Can you work these out from the model? Positions are in its coordinate system, mm. Give positions to 0.01 mm unless a question says otherwise; leave off trailing zeros. Write each loop counter-clockwise with the first axis right and the second up, starting at its lowest first coordinate (ties: lowest second). Pieces come first, ordered by that corner, then holes.
1. I'm going to push flat-ended pins straight in: pin 1 (1 mm diameter, centred on x = -2, y = 93, fed in from +Z); pin 2 (3 mm diameter, centred on x = -0.5, z = -43, fed in from +Y); pin 3 (2.5 mm diameter, centred on y = 149.03, z = 29.78, fed in from -X); pin 4 (3 mm diameter, centred on x = -1.5, y = 119, fed in from -Z). Where does each tip first touch, or does it pass through?
2. Suppose I cut it at B-B (y = 93). Please give me the cut outline in (x, z) (3 decimals), and give its area (3 significant figures).
3. Suppose I cut it at A-A (z = -14). Please give me the cut outline in (x, y) (3 decimals), and give its area (3 significant figures).
4. Suppose I cut it at C-C (y = 42). Please give me the cut outline in (x, z) (3 decimals).
5. If I drill on probe 1 along Y at (x, z) = (-1, 27); probe 2 along Y at (x, z) = (-0.75, 7); probe 3 along Y at (x, z) = (-2, 44), over which ranges is the centre line in solid material (lowest first)?
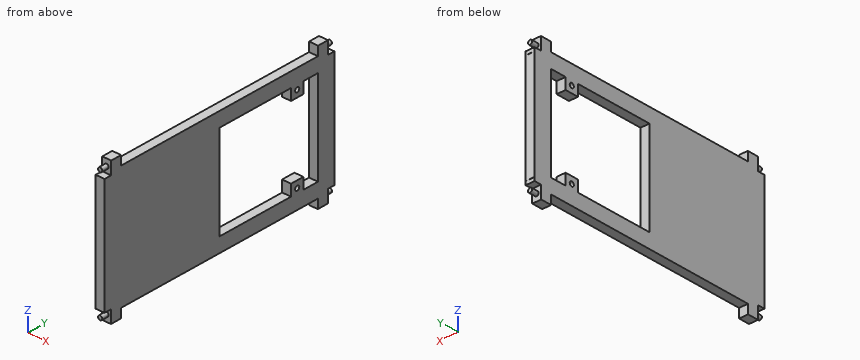
```python
from build123d import *

# Parameters (mm, degrees)
SKETCH1_R               = 49.53
SKETCH1_R_2             = 38.1
BOSS_EXTRUDE1_DEPTH     = 12.7
SKETCH4_W               = 6.35
SKETCH4_H               = 10.16
BOSS_EXTRUDE4_DEPTH     = 152.4
SKETCH6_R               = 49.53
BOSS_EXTRUDE8_DEPTH     = 12.7
CUT_EXTRUDE1_DEPTH      = 192.10018786
CUT_EXTRUDE1_DEPTH_BACK = 192.10018786
SKETCH8_W               = 6.35
SKETCH8_H               = 9.525
BOSS_EXTRUDE9_DEPTH     = 7.874
SKETCH9_R               = 1.5875
CUT_EXTRUDE2_DEPTH      = 192.831674819
SKETCH10_W              = 182.98458546
SKETCH10_H              = 212.101714012
CUT_EXTRUDE3_DEPTH      = 192.831674819
SKETCH13_W              = 128.016671202
SKETCH13_H              = 210.018995068
CUT_EXTRUDE4_DEPTH      = 191.199216379
SKETCH14_W              = 6.35
SKETCH14_H              = 8.918129625
SKETCH14_R              = 1.5
CUT_EXTRUDE5_DEPTH      = 5
SKETCH15_W              = 8.919843596
SKETCH15_H              = 5.203541281
CUT_EXTRUDE6_DEPTH      = 5
MIRROR4_COPY_1_SKETCH_W = 6.35
MIRROR4_COPY_1_SKETCH_H = 8.918129625
MIRROR4_COPY_1_SKETCH_R = 1.5
MIRROR4_COPY_1_DEPTH    = 5
MIRROR4_COPY_2_SKETCH_W = 8.919843596
MIRROR4_COPY_2_SKETCH_H = 5.203541281
MIRROR4_COPY_2_DEPTH    = 5
SKETCH16_W              = 6.35
SKETCH16_H              = 65.7800056
BOSS_EXTRUDE10_DEPTH    = 76.2


with BuildPart() as part:
    # Sketch1 → Boss-Extrude1 (new body)
    # profile 1 of 2: a face of its own
    with BuildSketch(Plane(origin=(0, 0, 0), x_dir=(1, 0, 0), z_dir=(0, 1, 0))):
        with Locations(Location((0, 0, 0), (0, 0, 270))):
            Circle(SKETCH1_R)
        Circle(SKETCH1_R_2, mode=Mode.SUBTRACT)
    # profile 2 of 2: a face of its own
    with BuildSketch(Plane(origin=(0, 0, 0), x_dir=(1, 0, 0), z_dir=(0, 1, 0))):
        with BuildLine():
            Line((-3.175, 37.967477859), (-3.175, -37.967477859))
            ThreePointArc((-3.175, -37.967477859), (0, -38.1), (3.175, -37.967477859))
            Line((3.175, -37.967477859), (3.175, 37.967477859))
            ThreePointArc((3.175, 37.967477859), (0, 38.1), (-3.175, 37.967477859))
        make_face()
    extrude(amount=BOSS_EXTRUDE1_DEPTH)

    # Sketch4 → Boss-Extrude4 (add)
    with BuildSketch(Plane(origin=(0, 12.7, 0), x_dir=(1, 0, 0), z_dir=(0, 1, 0))):
        with Locations((0, -37.9700028)):
            Rectangle(SKETCH4_W, SKETCH4_H)
        with Locations((0, 37.9700028)):
            Rectangle(SKETCH4_W, SKETCH4_H)
    extrude(amount=BOSS_EXTRUDE4_DEPTH)

    # Sketch6 → Boss-Extrude8 (add)
    with BuildSketch(Plane(origin=(0, 165.1, 0), x_dir=(1, 0, 0), z_dir=(0, 1, 0))):
        with Locations(Location((0, 0, 0), (0, 0, 270))):
            Circle(SKETCH6_R)
        with BuildLine():
            Line((-3.144660136, -37.9700028), (3.144660136, -37.9700028))
            ThreePointArc((3.144660136, -37.9700028), (0, -38.1), (-3.144660136, -37.9700028))
        make_face(mode=Mode.SUBTRACT)
        with BuildLine():
            Line((3.175, -37.967477859), (3.175, 37.967477859))
            ThreePointArc((3.175, 37.967477859), (38.1, 0), (3.175, -37.967477859))
        make_face(mode=Mode.SUBTRACT)
        with BuildLine():
            Line((3.144660136, 37.9700028), (-3.144660136, 37.9700028))
            ThreePointArc((-3.144660136, 37.9700028), (0, 38.1), (3.144660136, 37.9700028))
        make_face(mode=Mode.SUBTRACT)
        with BuildLine():
            Line((-3.175, 37.967477859), (-3.175, -37.967477859))
            ThreePointArc((-3.175, -37.967477859), (-38.1, 0), (-3.175, 37.967477859))
        make_face(mode=Mode.SUBTRACT)
    extrude(amount=BOSS_EXTRUDE8_DEPTH)

    # Sketch7 → Cut-Extrude1 (cut, two sides: drawn at the far end of the back side and taken through both)
    with BuildSketch(Plane.XZ.offset(-CUT_EXTRUDE1_DEPTH_BACK)):
        with BuildLine():
            Line((-49.106263984, -6.464962301), (-40.292319166, -5.304584452))
            ThreePointArc((-40.292319166, -5.304584452), (-40.64, 0), (-40.292319166, 5.304584452))
            Line((-40.292319166, 5.304584452), (-49.106263984, 6.464962301))
            ThreePointArc((-49.106263984, 6.464962301), (-49.53, 0), (-49.106263984, -6.464962301))
        make_face()
        with BuildLine():
            Line((40.292319166, -5.304584452), (49.106263984, -6.464962301))
            ThreePointArc((49.106263984, -6.464962301), (49.423952468, -3.239416991), (49.53, 0))
            ThreePointArc((49.53, 0), (49.423952468, 3.239416991), (49.106263984, 6.464962301))
            Line((49.106263984, 6.464962301), (40.292319166, 5.304584452))
            ThreePointArc((40.292319166, 5.304584452), (40.64, 0), (40.292319166, -5.304584452))
        make_face()
        with BuildLine():
            Line((37.774049218, -4.973047924), (40.292319166, -5.304584452))
            ThreePointArc((40.292319166, -5.304584452), (40.64, 0), (40.292319166, 5.304584452))
            Line((40.292319166, 5.304584452), (37.774049218, 4.973047924))
            ThreePointArc((37.774049218, 4.973047924), (38.1, 0), (37.774049218, -4.973047924))
        make_face()
        with BuildLine():
            Line((-40.292319166, -5.304584452), (-37.774049218, -4.973047924))
            ThreePointArc((-37.774049218, -4.973047924), (-38.1, 0), (-37.774049218, 4.973047924))
            Line((-37.774049218, 4.973047924), (-40.292319166, 5.304584452))
            ThreePointArc((-40.292319166, 5.304584452), (-40.64, 0), (-40.292319166, -5.304584452))
        make_face()
    extrude(amount=CUT_EXTRUDE1_DEPTH + CUT_EXTRUDE1_DEPTH_BACK, mode=Mode.SUBTRACT)

    # Sketch8 → Boss-Extrude9 (add)
    with BuildSketch(Plane.XY.offset(-32.8900028)):
        with Locations((0, 28.7655)):
            Rectangle(SKETCH8_W, SKETCH8_H)
        with Locations((0, 149.0345)):
            Rectangle(SKETCH8_W, SKETCH8_H)
    boss_extrude9 = extrude(amount=BOSS_EXTRUDE9_DEPTH)

    # Mirror1: Boss-Extrude9 across plane
    add(boss_extrude9.mirror(Plane.XY.offset(0.0029972)))

    # Sketch9 → Cut-Extrude2 (cut, through all)
    with BuildSketch(Plane(origin=(3.175, 0, 0), x_dir=(0, 0, -1), z_dir=(1, 0, 0))):
        with Locations((29.7785028, 28.7655)):
            Circle(SKETCH9_R)
        with Locations((29.7785028, 149.0345)):
            Circle(SKETCH9_R)
    cut_extrude2 = extrude(amount=-CUT_EXTRUDE2_DEPTH, mode=Mode.SUBTRACT)

    # Mirror2: Cut-Extrude2 across plane
    add(cut_extrude2.mirror(Plane.XY.offset(0.0029972)), mode=Mode.SUBTRACT)

    # Sketch10 → Cut-Extrude3 (cut, through all)
    with BuildSketch(Plane.ZY.offset(3.175)):
        with Locations((0.893156514, 95.768616586)):
            Rectangle(SKETCH10_W, SKETCH10_H)
    extrude(amount=CUT_EXTRUDE3_DEPTH, mode=Mode.SUBTRACT)

    # Sketch13 → Cut-Extrude4 (cut, through all)
    with BuildSketch(Plane(origin=(3.175, 0, 0), x_dir=(0, 0, -1), z_dir=(1, 0, 0))):
        with Locations((3.230681638, 97.01833452)):
            Rectangle(SKETCH13_W, SKETCH13_H)
    extrude(amount=CUT_EXTRUDE4_DEPTH, mode=Mode.SUBTRACT)

    # Sketch14 → Cut-Extrude5 (cut)
    with BuildSketch(Plane(origin=(0, 177.8, 0), x_dir=(1, 0, 0), z_dir=(0, 1, 0))):
        with Locations((0, 44.969067612)):
            Rectangle(SKETCH14_W, SKETCH14_H)
        with Locations(Location((0.015169932, 44.788132425, 0), (0, 0, 270))):
            Circle(SKETCH14_R, mode=Mode.SUBTRACT)
    cut_extrude5 = extrude(amount=-CUT_EXTRUDE5_DEPTH, mode=Mode.SUBTRACT)

    # Sketch15 → Cut-Extrude6 (cut)
    with BuildSketch(Plane(origin=(0, 172.8, 0), x_dir=(1, 0, 0), z_dir=(0, 1, 0))):
        with Locations((0.161262395, 49.49484543)):
            Rectangle(SKETCH15_W, SKETCH15_H)
    cut_extrude6 = extrude(amount=CUT_EXTRUDE6_DEPTH, mode=Mode.SUBTRACT)

    # Mirror3: Cut-Extrude5, Cut-Extrude6 across plane
    add(cut_extrude5.mirror(Plane.XY.offset(0.0029972)), mode=Mode.SUBTRACT)
    add(cut_extrude6.mirror(Plane.XY.offset(0.0029972)), mode=Mode.SUBTRACT)

    # Mirror4: Cut-Extrude5, Cut-Extrude6 across plane
    add(cut_extrude5.mirror(Plane(origin=(0, 88.9, 0), x_dir=(0, 0, 1), z_dir=(0, -1, 0))), mode=Mode.SUBTRACT)
    add(cut_extrude6.mirror(Plane(origin=(0, 88.9, 0), x_dir=(0, 0, 1), z_dir=(0, -1, 0))), mode=Mode.SUBTRACT)

    # Mirror4 copy 1 sketch → Mirror4 copy 1 (cut)
    with BuildSketch(Plane(origin=(0, 0, 0.0059944), x_dir=(1, 0, 0), z_dir=(0, -1, 0))):
        with Locations((0, 44.969067612)):
            Rectangle(MIRROR4_COPY_1_SKETCH_W, MIRROR4_COPY_1_SKETCH_H)
        with Locations(Location((0.015169932, 44.788132425, 0), (0, 0, 270))):
            Circle(MIRROR4_COPY_1_SKETCH_R, mode=Mode.SUBTRACT)
    extrude(amount=-MIRROR4_COPY_1_DEPTH, mode=Mode.SUBTRACT)

    # Mirror4 copy 2 sketch → Mirror4 copy 2 (cut)
    with BuildSketch(Plane(origin=(0, 5, 0.0059944), x_dir=(1, 0, 0), z_dir=(0, -1, 0))):
        with Locations((0.161262395, 49.49484543)):
            Rectangle(MIRROR4_COPY_2_SKETCH_W, MIRROR4_COPY_2_SKETCH_H)
    extrude(amount=MIRROR4_COPY_2_DEPTH, mode=Mode.SUBTRACT)

    # Sketch16 → Boss-Extrude10 (add)
    with BuildSketch(Plane(origin=(0, 12.7, 0), x_dir=(1, 0, 0), z_dir=(0, 1, 0))):
        Rectangle(SKETCH16_W, SKETCH16_H)
    extrude(amount=BOSS_EXTRUDE10_DEPTH)


solid = part.part
```
Checks:
1. pin 1: stops at z = 43.05
1. pin 2: stops at y = 177.8
1. pin 3: passes through
1. pin 4: stops at z = -43.05
2. outline: (-3.175, -43.05) - (3.175, -43.05) - (3.175, -32.89) - (-3.175, -32.89) - close; (-3.175, 32.89) - (3.175, 32.89) - (3.175, 43.05) - (-3.175, 43.05) - close
2. area: 129 mm2
3. outline: (-3.175, 0) - (3.175, 0) - (3.175, 88.9) - (-3.175, 88.9) - close; (-3.175, 165.1) - (3.175, 165.1) - (3.175, 177.8) - (-3.175, 177.8) - close
3. area: 645 mm2
4. outline: (-3.175, -43.05) - (3.175, -43.05) - (3.175, 43.05) - (-3.175, 43.05) - close
5. probe 1: y = 0 to 88.9, 144.27 to 153.8, 165.1 to 177.8
5. probe 2: y = 0 to 88.9, 165.1 to 177.8
5. probe 3: y = 5 to 12.7, 165.1 to 172.8
